The figure shows three views and two pictorial views of one solid part (mm, origin at its lowest corner). Answer the questions. A direction names the side the tool comes from. Give positions to 0.01 mm unless a question says otherwise; leave off trailing zeros. Order: outer loops, then holes, each group sorted by start corner. A loop starts at its lowest first (then second) coordinate and runs counter-clockwise, first axis right, second up. Notation, with made-up numbers: (-17, 45.5) - (39, 45.5) arc R24 cw to (39, 72.5) - close; hole circle Ø4 at (4, 28.5). An arc over 180 degrees is marked (long way). Write item = value, one per line.
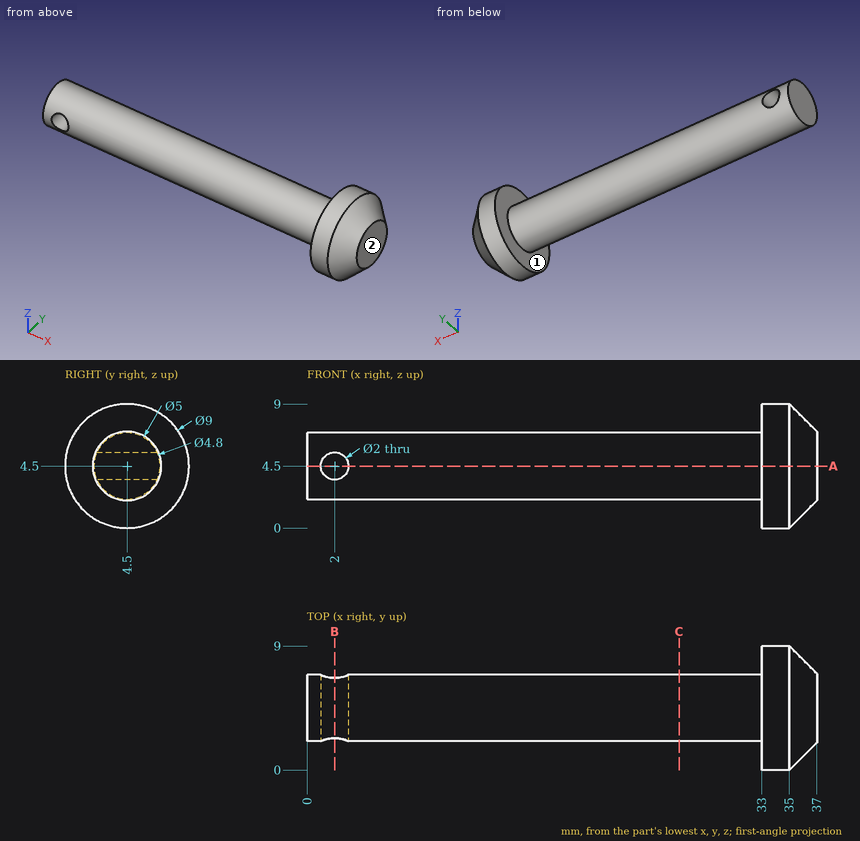
1. For the marked faces 1 and 2, determine the directions among +Z, -Z, +X, -X, +Y, -Y from which every point of the face is accessible in a straight line to the end or side of a thin tool.
Recorded:
face_1 = -X
face_2 = +Z, -Z, +X, +Y, -Y
2. Flat-ended cylindrical pins translate along their axes: pin 1 (1.2 mm diameter, centred on x = 2, z = 4.5, fed in from +Y); pin 2 (2 mm diameter, centred on y = 8, z = 3.5, fed in from +X); pin 3 (1.5 mm diameter, centred on x = 6, z = 4.5, fed in from +Y); pin 4 (1.5 mm diameter, centred on x = 4, y = 3.5, fed in from +Z). Find the tip coordinate at first contact, or state that the pin passes through.
Recorded:
pin_1 = through
pin_2 = 36.86
pin_3 = 6.9
pin_4 = 6.89
3. Section B-B (x = 2) is taken. Determine the outline of the cut face in (y, z).
Recorded:
outline = (2.32, 3.5) arc R2.4 ccw to (6.68, 3.5) - close; (2.32, 5.5) - (6.68, 5.5) arc R2.4 ccw to start
4. Section A-A (z = 4.5) is taken. Determine the outline of the cut face in (x, y), and give its area (3 significant figures).
Recorded:
outline = (0, 2.1) - (1, 2.1) - (1, 6.9) - (0, 6.9) - close; (3, 2.1) - (33, 2.1) - (33, 0) - (35, 0) - (37, 2) - (37, 7) - (35, 9) - (33, 9) - (33, 6.9) - (3, 6.9) - close
area = 181 mm^2
5. Section C-C (x = 27) is taken. Determine the outline of the cut face in (y, z).
Recorded:
outline = circle Ø4.8 at (4.5, 4.5)
6. Straight lines are drawn through the part: L1, parallel to X at y = 5.4, z = 4.5; L2, parallel to X at y = 5.25, z = 4; L3, parallel to Z at x = 34.5, y = 4. For each, find the intervals that lie inside material, in ascending order. Write a range as [from, to].
Recorded:
L1 = [0, 1], [3, 37]
L2 = [0, 1.13], [2.87, 37]
L3 = [0.03, 8.97]
